Geometry check sheet. Reference: drawing and pictorial views, mm from the part's lowest x, y, z. A direction names the side the tool comes from. Round coordinates to 2 decimals unless told otherwise and drop trailing zeros. Write each loop counter-clockwise with the first axis right and the second up, starting at its lowest first coordinate (ties: lowest second). Pieces come first, ordered by that corner, then holes. Notation, with made-up numbers: (-28, 15.25) - (-20, 15.25) arc R23 ccw to (-20, 49.25) - close; hole circle Ø10 at (6.25, -22). An arc over 180 degrees is marked (long way). Return JSON: item names as keys, results as strings.
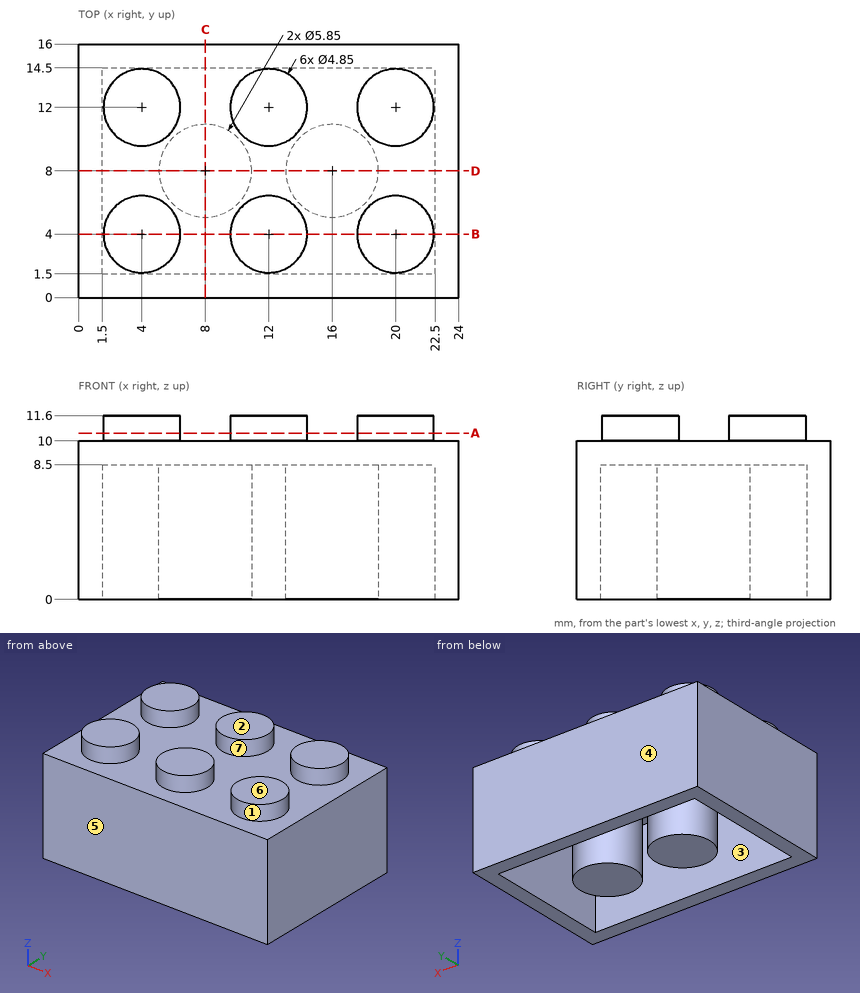
(1) Section check D-D, the plane y = 8. Enter the section's corners in (x, z) (3 decimals).
Response values:
{"outline": "(0, 0) - (1.5, 0) - (1.5, 8.5) - (5.075, 8.5) - (5.075, 0) - (10.925, 0) - (10.925, 8.5) - (13.075, 8.5) - (13.075, 0) - (18.925, 0) - (18.925, 8.5) - (22.5, 8.5) - (22.5, 0) - (24, 0) - (24, 10) - (0, 10) - close"}
(2) Material ranges on line 1 along Y through (x, z) = (2, 6.75); line 2 along X through (y, z) = (1.75, 5.5); line 3 along X through (y, z) = (5.5, 1.5), recorded low to high. Write a range as [from, to].
Response values:
{"line 1": "y = [0, 1.5], [14.5, 16]", "line 2": "x = [0, 1.5], [22.5, 24]", "line 3": "x = [0, 1.5], [6.48, 9.52], [14.48, 17.52], [22.5, 24]"}
(3) Release check for a two-part mould opening along Y. For the marked faces 4, 5, 6 and 7 record: pulls with the +Y half, pulls with the -Y half, needs draft (parallel to the pull), parting line crosses it, or undercut.
Response values:
{"face 4": "pulls with the +Y half", "face 5": "pulls with the -Y half", "face 6": "needs draft", "face 7": "undercut"}
(4) Section check B-B, the plane y = 4. Enter the section's corners in (x, z) (3 decimals), plus the area to 3 significant figures.
Response values:
{"outline": "(0, 0) - (1.5, 0) - (1.5, 8.5) - (22.5, 8.5) - (22.5, 0) - (24, 0) - (24, 10) - (22.425, 10) - (22.425, 11.6) - (17.575, 11.6) - (17.575, 10) - (14.425, 10) - (14.425, 11.6) - (9.575, 11.6) - (9.575, 10) - (6.425, 10) - (6.425, 11.6) - (1.575, 11.6) - (1.575, 10) - (0, 10) - close", "area": "84.8 mm^2"}
(5) Access from +Z, -Z, +X, -X, +Y, -Y to the whole of each face (thin tool, end or side, straight path). Record for the marked faces 1, 2 and 3.
Response values:
{"face 1": "+Z", "face 2": "+Z, +X, -X, +Y, -Y", "face 3": "-Z"}
(6) Section check A-A, the plane z = 10.5. Enter the section's corners in (x, y) (3 decimals).
Response values:
{"outline": "circle Ø4.85 at (4, 4); circle Ø4.85 at (4, 12); circle Ø4.85 at (12, 4); circle Ø4.85 at (12, 12); circle Ø4.85 at (20, 4); circle Ø4.85 at (20, 12)"}
(7) Section check C-C, the plane x = 8. Enter the section's corners in (y, z) (3 decimals).
Response values:
{"outline": "(0, 0) - (1.5, 0) - (1.5, 8.5) - (5.075, 8.5) - (5.075, 0) - (10.925, 0) - (10.925, 8.5) - (14.5, 8.5) - (14.5, 0) - (16, 0) - (16, 10) - (0, 10) - close"}
